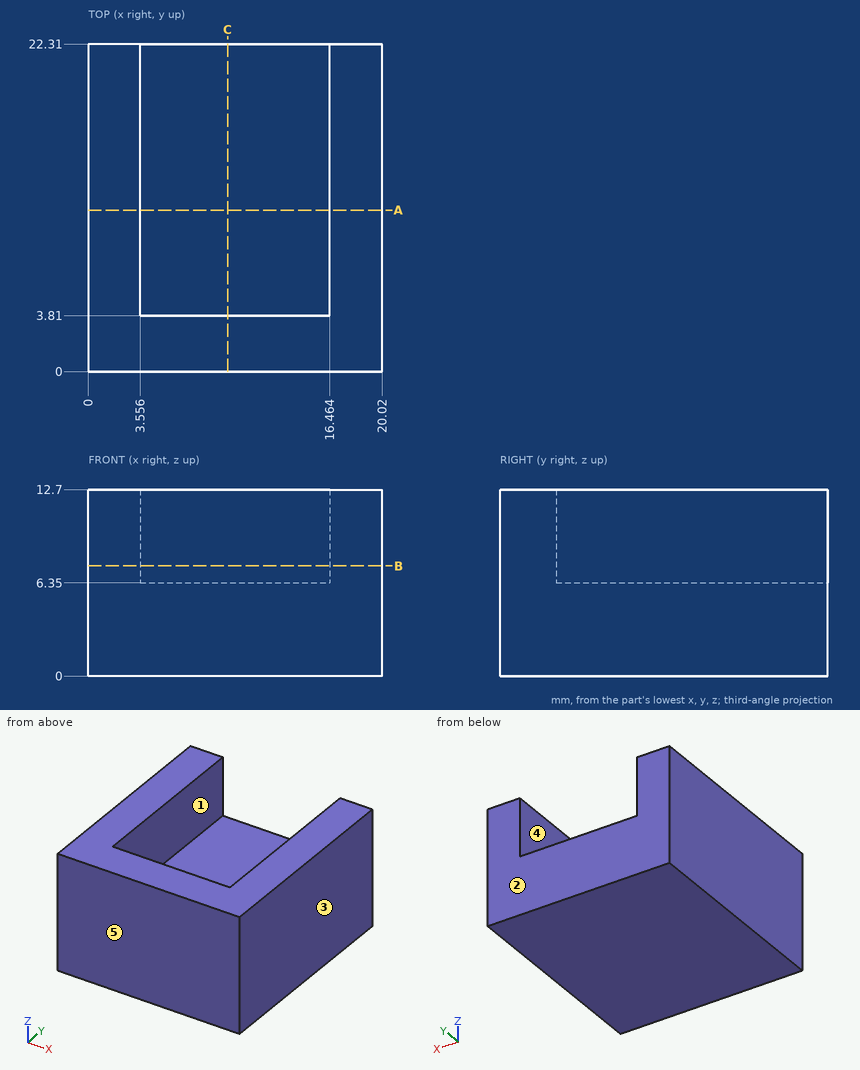
Drawing for the job (mm, zero at the part's lowest x, y, z). A direction names the side the tool comes from. Round coordinates to 2 decimals unless told otherwise and drop trailing zeros. Order: outer loops, then holes, each group sorted by start corner. A loop starts at its lowest first (then second) coordinate and runs counter-clockwise, first axis right, second up.
Item 1: Probe line 1 along X through (y, z) = (21.25, 8.5); line 2 along Y through (x, z) = (10, 9.5); line 3 along Z through (x, y) = (6.25, 6.25). List the from-to ranges inside material, lowest first.
Item 2: Tool access for the marked faces 4 and 5: list every direction of +Z, -Z, +X, -X, +Y, -Y with a clear straight run to the whole face (end or side of a thin tool).
Item 3: Mould opens along X. For the marked faces 1, 2 and 3 say: pulls with the +X half, pulls with the -X half, needs draft (parallel to the pull), parting line crosses it, or undercut.
Item 4: Pin check, flat tips, straight feed: pin 1 (4 mm diameter, centred on x = 9, y = 9, fed in from +Z); pin 2 (3 mm diameter, centred on x = 10, z = 8, fed in from +Y). Stop position of each tip, or through.
Item 5: Saw through at B-B on z = 7.5. Write the cut outline in (x, y).
Item 6: Saw through at C-C on x = 9.5. Write the cut outline in (y, z).
Item 7: Saw through at A-A on y = 11. Write the cut outline in (x, z).
Reported:
1. line 1: x = 0 to 3.56, 16.46 to 20.02
1. line 2: y = 0 to 3.81
1. line 3: z = 0 to 6.35
2. face 4: +Z, +Y
2. face 5: +Z, -Z, +X, -X, -Y
3. face 1: undercut
3. face 2: needs draft
3. face 3: pulls with the +X half
4. pin 1: stops at z = 6.35
4. pin 2: stops at y = 3.81
5. outline: (0, 0) - (20.02, 0) - (20.02, 22.31) - (16.46, 22.31) - (16.46, 3.81) - (3.56, 3.81) - (3.56, 22.31) - (0, 22.31) - close
6. outline: (0, 0) - (22.31, 0) - (22.31, 6.35) - (3.81, 6.35) - (3.81, 12.7) - (0, 12.7) - close
7. outline: (0, 0) - (20.02, 0) - (20.02, 12.7) - (16.46, 12.7) - (16.46, 6.35) - (3.56, 6.35) - (3.56, 12.7) - (0, 12.7) - close
